from build123d import *

# Parameters (mm, degrees)
F0_W     = 1422.4
F0_H     = 558.8
F0_W_2   = 558.8
F1_DEPTH = 762
F2_W     = 1422.4
F2_H     = 609.6
F3_DEPTH = 558.8


with BuildPart() as f1:
    # F0 (on Top) → F1 (new body)
    with BuildSketch(Plane.XY):
        Rectangle(F0_W, F0_H)
        with Locations((990.6, 0)):
            Rectangle(F0_W_2, F0_H)
    extrude(amount=F1_DEPTH)

    # F2 (on face) → F3 (cut)
    with BuildSketch(Plane.XZ.offset(279.4)):
        with Locations((0, 304.8)):
            Rectangle(F2_W, F2_H)
    extrude(amount=-F3_DEPTH, mode=Mode.SUBTRACT)


solid = f1.part
Can you work these out from the model? Positions are in its coordinate system, mm. A direction names the side the tool comes from. Give positions to 0.01 mm unless a question says otherwise; leave off trailing zeros. Loops run counter-clockwise (first coordinate to the right, second up) from the corner with the lowest first, then second, coordinate; pieces in that order, holes last. Notation, with made-up numbers: (49, 6) -> (71, 6) arc R24 cw to (71, 23) -> close; hole circle Ø6 at (52, 11.25). An arc over 180 degrees is marked (long way). Use one line per item in the form item = value.
1) If we section it at A-A (y = 91.5): Please give me the cut outline in (x, z), plus the area to 3 significant figures.
Answers:
outline = (-711.2, 609.6) -> (711.2, 609.6) -> (711.2, 0) -> (1270, 0) -> (1270, 762) -> (-711.2, 762) -> close
area = 643,000 mm²
2) If we section it at C-C (z = 549.5): Please give me the cut outline in (x, y).
Answers:
outline = (711.2, -279.4) -> (1270, -279.4) -> (1270, 279.4) -> (711.2, 279.4) -> close
3) If we section it at B-B (x = -238): Please give me the cut outline in (y, z), plus the area to 3 significant figures.
Answers:
outline = (-279.4, 609.6) -> (279.4, 609.6) -> (279.4, 762) -> (-279.4, 762) -> close
area = 85,200 mm²
4) For faces 1 (the face through (-10, -4, 609.6)), 2 (the face through (706, -279.4, 630)), which set-ups out of +Z, -Z, +X, -X, +Y, -Y let a thin tool reach every point of the face, with its end or its side?
Answers:
face_1 = -Z, -X, +Y, -Y
face_2 = +Z, -Z, +X, -X, -Y
5) Will these pins go through, and if not, where does the flat tip stop? pin 1 (6 mm diameter, centred on y = -220, z = 340, fed in from -X); pin 2 (5 mm diameter, centred on x = 131, y = 128, fed in from -Z).
Answers:
pin_1 = 711.2
pin_2 = 609.6
6) I need wall thicknesses on line 1 along X through (y, z) = (-68, 602.5); line 2 along Z through (x, y) = (466, 230). Which ranges of each line are inside material? Lowest first, please.
Answers:
line_1 = 711.2 to 1270
line_2 = 609.6 to 762
